CAD build for the part. Positions are in the model's coordinates, mm. A direction names the side the tool comes from. Round coordinates to 2 decimals unless told otherwise and drop trailing zeros. Write each loop counter-clockwise with the first axis right and the second up, starting at its lowest first coordinate (ties: lowest second). Pieces come first, ordered by that corner, then holes. Notation, with made-up numbers: M -18,4.5 L 33,4.5 A20 ccw 33,21.5 Z; hole C 50,33 d11. An arc over 180 degrees is marked long. Write each question's results on one line, items separated by ' | '. Start each with the question number.
```python
from build123d import *

# Parameters (mm, degrees)
SKETCH3_W                                           = 152
SKETCH3_H                                           = 125
BOSS_EXTRUDE2_DEPTH                                 = 10
KES_EKSTR_ZYON1_DEPTH                               = 3
CBORE_FOR_M5_HEX_SOCKET_HEAD_CAP_SCREW1_D           = 5.8
CBORE_FOR_M5_HEX_SOCKET_HEAD_CAP_SCREW1_DEPTH       = 15
CBORE_FOR_M5_HEX_SOCKET_HEAD_CAP_SCREW1_CBORE_D     = 9
CBORE_FOR_M5_HEX_SOCKET_HEAD_CAP_SCREW1_CBORE_DEPTH = 5.5
CBORE_FOR_M5_HEX_SOCKET_HEAD_CAP_SCREW1_TIP         = 1.742495795
CBORE_FOR_M5_HEX_SOCKET_HEAD_CAP_SCREW2_D           = 5.5
CBORE_FOR_M5_HEX_SOCKET_HEAD_CAP_SCREW2_CBORE_D     = 10
CBORE_FOR_M5_HEX_SOCKET_HEAD_CAP_SCREW2_CBORE_DEPTH = 5.4
CBORE_FOR_M4_HEX_SOCKET_HEAD_CAP_SCREW2_D           = 4.5
CBORE_FOR_M4_HEX_SOCKET_HEAD_CAP_SCREW2_CBORE_D     = 8
CBORE_FOR_M4_HEX_SOCKET_HEAD_CAP_SCREW2_CBORE_DEPTH = 4.4
SKETCH13_W                                          = 40
SKETCH13_H                                          = 30
CUT_EXTRUDE1_DEPTH                                  = 5
SKETCH14_W                                          = 15
SKETCH14_H                                          = 5
BOSS_EXTRUDE3_DEPTH                                 = 152


with BuildPart() as part:
    # Sketch3 → Boss-Extrude2 (new body)
    with BuildSketch(Plane.XY):
        Rectangle(SKETCH3_W, SKETCH3_H)
    extrude(amount=BOSS_EXTRUDE2_DEPTH)

    # Çizim2 → Kes-Ekstrüzyon1 (cut)
    with BuildSketch(Plane.XY.offset(10)):
        with BuildLine():
            Line((-34.5, -31), (-65.5, -31))
            ThreePointArc((-65.5, -31), (-71.156854249, -28.656854249), (-73.5, -23))
            Line((-73.5, -23), (-73.5, 23))
            ThreePointArc((-73.5, 23), (-71.156854249, 28.656854249), (-65.5, 31))
            Line((-65.5, 31), (-34.5, 31))
            ThreePointArc((-34.5, 31), (-28.843145751, 28.656854249), (-26.5, 23))
            Line((-26.5, 23), (-26.5, -23))
            ThreePointArc((-26.5, -23), (-28.843145751, -28.656854249), (-34.5, -31))
        make_face()
        with BuildLine():
            Line((65.5, -31), (34.5, -31))
            ThreePointArc((34.5, -31), (28.843145751, -28.656854249), (26.5, -23))
            Line((26.5, -23), (26.5, 23))
            ThreePointArc((26.5, 23), (28.843145751, 28.656854249), (34.5, 31))
            Line((34.5, 31), (65.5, 31))
            ThreePointArc((65.5, 31), (71.156854249, 28.656854249), (73.5, 23))
            Line((73.5, 23), (73.5, -23))
            ThreePointArc((73.5, -23), (71.156854249, -28.656854249), (65.5, -31))
        make_face()
    extrude(amount=-KES_EKSTR_ZYON1_DEPTH, mode=Mode.SUBTRACT)

    # CBORE for M5 Hex Socket Head Cap Screw1
    with Locations(Plane.XY.offset(10)):
        with Locations((-12, 30), (12, 30), (-12, -45), (12, -45)):
            CounterBoreHole(CBORE_FOR_M5_HEX_SOCKET_HEAD_CAP_SCREW1_D / 2, CBORE_FOR_M5_HEX_SOCKET_HEAD_CAP_SCREW1_CBORE_D / 2, CBORE_FOR_M5_HEX_SOCKET_HEAD_CAP_SCREW1_CBORE_DEPTH, depth=CBORE_FOR_M5_HEX_SOCKET_HEAD_CAP_SCREW1_DEPTH)
            with Locations((0, 0, -(CBORE_FOR_M5_HEX_SOCKET_HEAD_CAP_SCREW1_DEPTH + CBORE_FOR_M5_HEX_SOCKET_HEAD_CAP_SCREW1_TIP / 2))):  # 118° drill point
                Cone(0, CBORE_FOR_M5_HEX_SOCKET_HEAD_CAP_SCREW1_D / 2, CBORE_FOR_M5_HEX_SOCKET_HEAD_CAP_SCREW1_TIP, mode=Mode.SUBTRACT)

    # CBORE for M5 Hex Socket Head Cap Screw2 (through all)
    with Locations(Plane(origin=(0, 0, 0), x_dir=(1, 0, 0), z_dir=(0, 0, -1))):
        with Locations((-69, -15), (-31, -15), (-69, 15), (-31, 15), (31, -15), (31, 15), (69, 15), (69, -15)):
            CounterBoreHole(CBORE_FOR_M5_HEX_SOCKET_HEAD_CAP_SCREW2_D / 2, CBORE_FOR_M5_HEX_SOCKET_HEAD_CAP_SCREW2_CBORE_D / 2, CBORE_FOR_M5_HEX_SOCKET_HEAD_CAP_SCREW2_CBORE_DEPTH)

    # CBORE for M4 Hex Socket Head Cap Screw2 (through all)
    with Locations(Plane(origin=(0, 0, 0), x_dir=(-1, 0, 0), z_dir=(0, 0, -1))):
        with Locations((-15, 7.5), (-15, -7.5), (15, 7.5), (15, -7.5)):
            CounterBoreHole(CBORE_FOR_M4_HEX_SOCKET_HEAD_CAP_SCREW2_D / 2, CBORE_FOR_M4_HEX_SOCKET_HEAD_CAP_SCREW2_CBORE_D / 2, CBORE_FOR_M4_HEX_SOCKET_HEAD_CAP_SCREW2_CBORE_DEPTH)

    # Sketch13 → Cut-Extrude1 (cut)
    with BuildSketch(Plane.XY.offset(10)):
        Rectangle(SKETCH13_W, SKETCH13_H)
    extrude(amount=-CUT_EXTRUDE1_DEPTH, mode=Mode.SUBTRACT)

    # Sketch14 → Boss-Extrude3 (add)
    with BuildSketch(Plane.ZY.offset(-76)):
        with Locations((2.5, -65)):
            Rectangle(SKETCH14_W, SKETCH14_H)
    extrude(amount=BOSS_EXTRUDE3_DEPTH)


solid = part.part
```
1) Saw through at C-C, the plane x = 31. Write the cut outline in (y, z).
2) 3-axis set-ups, long thin cutter, end or side, ignore diameter. For faces 4 (the face through (33.747, 14.879, 6.211)), 5 (the face through (0, -15, 8)), 6 (the face through (71.2, -12.8, 5.4)): which of +Z, -Z, +X, -X, +Y, -Y reach the whole face in a straight line?
3) Saw through at A-A, the plane y = -7.5. State how many separate pieces and enclosed holes the cut face has, plus the area to 3 significant figures.
4) Pull direction Y, two halves, no side cores. Call faces 1 (the face through (1, -67.5, 2)), 2 (the face through (-28.253, 14.879, 6.211)), 3 (the face through (1, -18, 10)): pulls with the +Y half, pulls with the -Y half, needs draft (parallel to the pull), parting line crosses it, or undercut.
5) Wall check: line 1 along Y through (x, z) = (-12, 5.65); line 2 along Y through (x, z) = (-31, 3.25); line 3 along X through (y, z) = (-16, 8.5). Give the ranges that are in metal, low to high. Write a range as from..to.
6) Saw through at D-D, the plane y = -35.5. Write the cut outline in (x, z).
7) Drop flat-ended pins along their axis: pin 1 Ø6.5 at (x, y) = (-31, 15) entering from -Z; pin 2 Ø8 at (x, y) = (-69, 15) entering from +Z; pin 3 Ø4 at (x, y) = (13.5, -6) entering from -Z. Give the stop position or say it passes through.
Filled sheet:
1) outline: M -67.5,-5 L -62.5,-5 L -62.5,0 L -20,0 L -20,5.4 L -17.75,5.4 L -17.75,7 L -30.19,7 L -30.19,10 L -67.5,10 Z; M -12.25,5.4 L -10,5.4 L -10,0 L 10,0 L 10,5.4 L 12.25,5.4 L 12.25,7 L -12.25,7 Z; M 17.75,5.4 L 20,5.4 L 20,0 L 62.5,0 L 62.5,10 L 30.19,10 L 30.19,7 L 17.75,7 Z
2) face 4: +Z, -Z | face 5: +Z | face 6: -Z
3) separate pieces: 3 | enclosed holes: 0 | area: 962 mm^2
4) face 1: pulls with the -Y half | face 2: undercut | face 3: needs draft
5) line 1: y = -67.5..-49.5, -40.5..-15, 15..25.5, 34.5..62.5 | line 2: y = -67.5..-20, -10..10, 20..62.5 | line 3: x = -76..-73.5, -26.5..26.5, 73.5..76
6) outline: M -76,0 L 76,0 L 76,10 L -76,10 Z
7) pin 1: stops at z = 5.4 | pin 2: stops at z = 7 | pin 3: stops at z = 0
